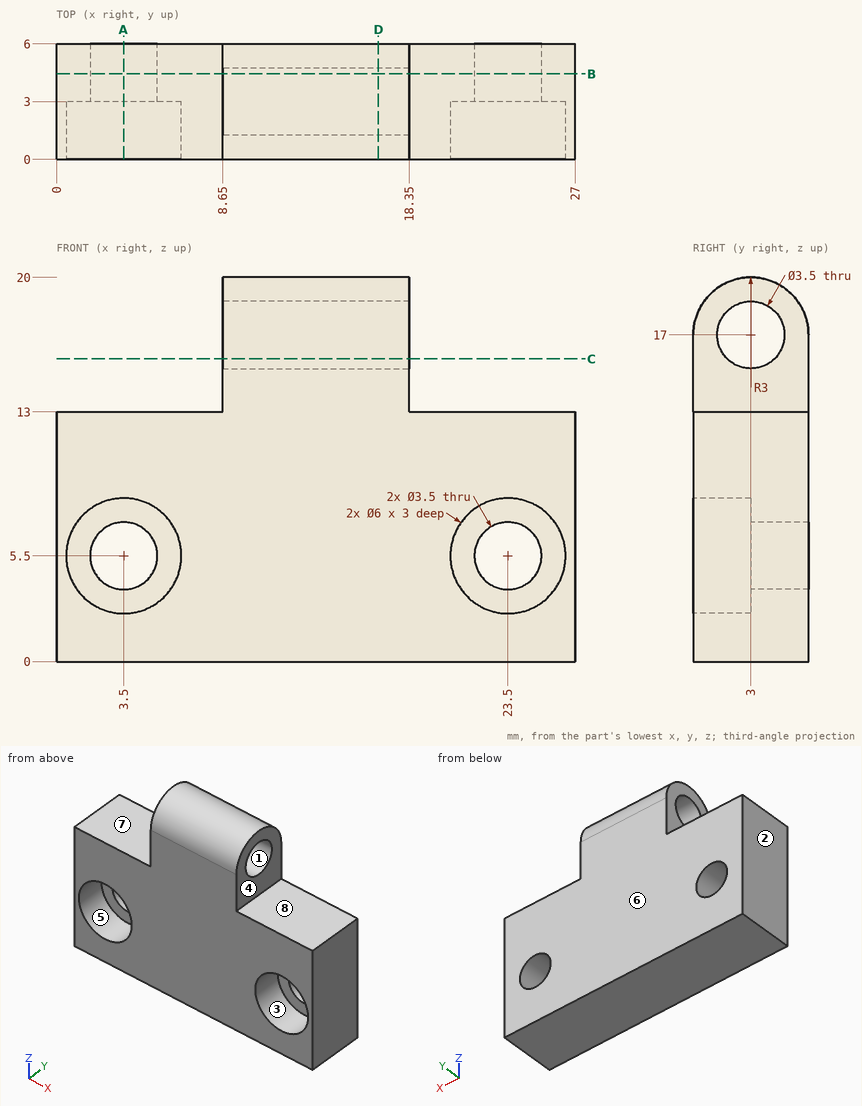
For this review, use the dimensioned drawing (mm, ordinates from the lowest corner) and the shaded views. A direction names the side the tool comes from. Give positions to 0.01 mm unless a question says otherwise; leave off trailing zeros. Order: outer loops, then holes, each group sorted by start corner. A loop starts at its lowest first (then second) coordinate and runs counter-clockwise, first axis right, second up. Notation, with made-up numbers: (47, 74.25) - (51, 74.25) arc R25 cw to (51, 100.25) - close; hole circle Ø8 at (85.5, 48.25). An arc over 180 degrees is marked (long way). Write item = value, one per line. Start each with the question number.
Q1. Tool access review of the marked faces 5, 6, 7 and 8: name each direction out of +Z, -Z, +X, -X, +Y, -Y from which nothing blocks a thin tool from reaching the whole face with its end or side.
Q2. We need section B-B on y = 4.45. State the section outline as (x, z) points, plus the area to 3 significant figures.
Q3. Mouldability with a two-part tool opening along X and no side actions: class the marked faces 1, 2, 3 and 4 as released by +X, released by -X, zero draft, split by the parting line, or undercut.
Q4. Clearance check with flat-ended pins moving along their axes: pin 1 Ø2 at (y, z) = (3.5, 2.5) entering from -X; pin 2 Ø4.5 at (x, z) = (23.5, 5.5) entering from -Y; pin 3 Ø3 at (x, y) = (23, 1.5) entering from +Z. State where each tip first meets the part, or that it passes through.
Q5. We need section D-D on x = 16.75. State the section outline as (y, z) points, plus the area to 3 significant figures.
Q6. To check wall thickness, follow L1, parallel to Z at x = 3.5, y = 1.4; L2, parallel to X at y = 1.8, z = 7.5; L3, parallel to Z at x = 3.5, y = 3.8. State the ranges of each line that lie inside material, in increasing order. Write a range as from..to.
Q7. We need section C-C on z = 15.75. State the section outline as (x, y) points, plus the area to 3 significant figures.
Q8. We need section A-A on x = 3.5. State the section outline as (y, z) points, plus the area to 3 significant figures.
Working result:
q1.face_5 = -Y
q1.face_6 = +Z, -Z, +X, -X, +Y
q1.face_7 = +Z, -X, +Y, -Y
q1.face_8 = +Z, +X, +Y, -Y
q2.outline = (0, 0) - (27, 0) - (27, 13) - (18.35, 13) - (18.35, 16.02) - (8.65, 16.02) - (8.65, 13) - (0, 13) - close; (8.65, 17.98) - (18.35, 17.98) - (18.35, 19.63) - (8.65, 19.63) - close; hole circle Ø3.5 at (3.5, 5.5); hole circle Ø3.5 at (23.5, 5.5)
q2.area = 377 mm²
q3.face_1 = zero draft
q3.face_2 = released by -X
q3.face_3 = undercut
q3.face_4 = released by +X
q4.pin_1 = 0
q4.pin_2 = 3
q4.pin_3 = 13
q5.outline = (0, 0) - (6, 0) - (6, 17) arc R3 ccw to (0, 17) - close; hole circle Ø3.5 at (3, 17)
q5.area = 107 mm²
q6.L1 = 0..2.5, 8.5..13
q6.L2 = 0..1.26, 5.74..21.26, 25.74..27
q6.L3 = 0..3.75, 7.25..13
q7.outline = (8.65, 0) - (18.35, 0) - (18.35, 1.78) - (8.65, 1.78) - close; (8.65, 4.22) - (18.35, 4.22) - (18.35, 6) - (8.65, 6) - close
q7.area = 34.4 mm²
q8.outline = (0, 0) - (6, 0) - (6, 3.75) - (3, 3.75) - (3, 2.5) - (0, 2.5) - close; (0, 8.5) - (3, 8.5) - (3, 7.25) - (6, 7.25) - (6, 13) - (0, 13) - close
q8.area = 49.5 mm²
